Can you work these out from the model? Positions are in its coordinate system, mm. Face numbers are marked on the shaded views. Coordinates: 2 decimals unless noted, no trailing zeros. Write each loop counter-clockwise with the first axis right and the second up, starting at its lowest first coordinate (ties: lowest second). Pieces come first, ordered by that corner, then holes. Notation, with made-up numbers: M -26,84 L 8,84 A8 cw 8,89 Z; hole C -13.75,53 d1. An arc over 180 degrees is marked long. Use one line per item in the form item = value. Start each with the question number.
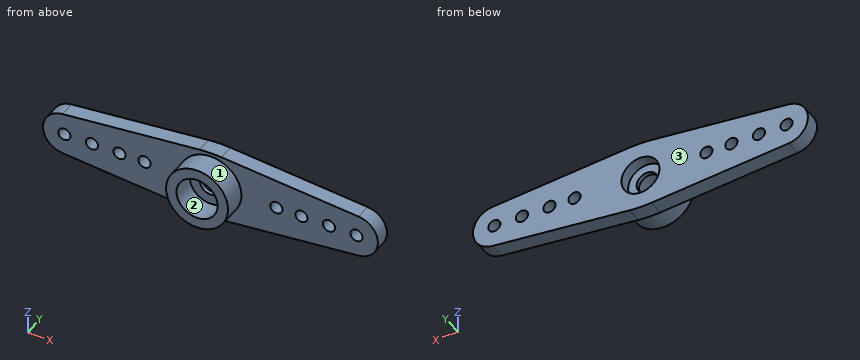
```python
from build123d import *

# Parameters (mm, degrees)
SKETCH1_R           = 3.3655
SKETCH1_R_2         = 2.2352
BOSS_EXTRUDE1_DEPTH = 2.54
SKETCH2_R           = 0.6604
SKETCH2_R_2         = 2.31775
SKETCH2_R_3         = 3.3655
SKETCH2_R_4         = 2.2352
SKETCH2_R_5         = 1.143
BOSS_EXTRUDE2_DEPTH = 1.7272
FILLET1_R           = 12.7
CUT_EXTRUDE1_START  = -1.27
SKETCH3_R           = 2.06375
SKETCH3_R_2         = 1.143
CUT_EXTRUDE1_DEPTH  = 1.27
SCALE1_SCALE        = 1.483924155


with BuildPart() as part:
    # Sketch1 → Boss-Extrude1 (new body)
    with BuildSketch(Plane(origin=(0, 0, 0), x_dir=(1, 0, 0), z_dir=(0, 1, 0))):
        with Locations(Location((0, 0, 0), (0, 0, 270))):
            Circle(SKETCH1_R)
        with Locations(Location((0, 0, 0), (0, 0, 270))):
            Circle(SKETCH1_R_2, mode=Mode.SUBTRACT)
    extrude(amount=BOSS_EXTRUDE1_DEPTH)

    # Sketch2 → Boss-Extrude2 (add)
    # profile 1 of 7: a face of its own
    with BuildSketch(Plane(origin=(0, 2.54, 0), x_dir=(1, 0, 0), z_dir=(0, 1, 0))):
        with BuildLine():
            ThreePointArc((-0.713521748, -3.755518873), (-3.8227, 0), (-0.713521748, 3.755518873))
            Line((-0.713521748, 3.755518873), (-16.092265178, 2.307544345))
            ThreePointArc((-16.092265178, 2.307544345), (-14.314807913, 1.713991165), (-13.55725, 0))
            ThreePointArc((-13.55725, 0), (-14.314807913, -1.713991165), (-16.092265178, -2.307544345))
            Line((-16.092265178, -2.307544345), (-0.713521748, -3.755518873))
        make_face()
        with Locations(Location((-12.8778, 0, 0), (0, 0, 270))):
            Circle(SKETCH2_R, mode=Mode.SUBTRACT)
        with Locations(Location((-9.8806, 0, 0), (0, 0, 270))):
            Circle(SKETCH2_R, mode=Mode.SUBTRACT)
        with Locations(Location((-7.1628, 0, 0), (0, 0, 270))):
            Circle(SKETCH2_R, mode=Mode.SUBTRACT)
    # profile 2 of 7: a face of its own
    with BuildSketch(Plane(origin=(0, 2.54, 0), x_dir=(1, 0, 0), z_dir=(0, 1, 0))):
        with Locations((-15.875, 0)):
            Circle(SKETCH2_R_2)
        with Locations(Location((-15.875, 0, 0), (0, 0, 270))):
            Circle(SKETCH2_R, mode=Mode.SUBTRACT)
    # profile 3 of 7: a face of its own
    with BuildSketch(Plane(origin=(0, 2.54, 0), x_dir=(1, 0, 0), z_dir=(0, 1, 0))):
        with BuildLine():
            Line((16.092265178, 2.307544345), (0.713521748, 3.755518873))
            ThreePointArc((0.713521748, 3.755518873), (2.944538578, 2.437771083), (3.8227, 0))
            ThreePointArc((3.8227, 0), (2.944538578, -2.437771083), (0.713521748, -3.755518873))
            Line((0.713521748, -3.755518873), (16.092265178, -2.307544345))
            ThreePointArc((16.092265178, -2.307544345), (13.55725, 0), (16.092265178, 2.307544345))
        make_face()
        with Locations(Location((7.1628, 0, 0), (0, 0, 270))):
            Circle(SKETCH2_R, mode=Mode.SUBTRACT)
        with Locations(Location((9.8806, 0, 0), (0, 0, 270))):
            Circle(SKETCH2_R, mode=Mode.SUBTRACT)
        with Locations(Location((12.8778, 0, 0), (0, 0, 270))):
            Circle(SKETCH2_R, mode=Mode.SUBTRACT)
    # profile 4 of 7: a face of its own
    with BuildSketch(Plane(origin=(0, 2.54, 0), x_dir=(1, 0, 0), z_dir=(0, 1, 0))):
        with Locations((15.875, 0)):
            Circle(SKETCH2_R_2)
        with Locations(Location((15.875, 0, 0), (0, 0, 270))):
            Circle(SKETCH2_R, mode=Mode.SUBTRACT)
    # profile 5 of 7: a face of its own
    with BuildSketch(Plane(origin=(0, 2.54, 0), x_dir=(1, 0, 0), z_dir=(0, 1, 0))):
        with BuildLine():
            Line((0.713521748, 3.755518873), (0, 3.8227))
            Line((0, 3.8227), (-0.713521748, 3.755518873))
            ThreePointArc((-0.713521748, 3.755518873), (-3.8227, 0), (-0.713521748, -3.755518873))
            Line((-0.713521748, -3.755518873), (0, -3.8227))
            Line((0, -3.8227), (0.713521748, -3.755518873))
            ThreePointArc((0.713521748, -3.755518873), (2.944538578, -2.437771083), (3.8227, 0))
            ThreePointArc((3.8227, 0), (2.944538578, 2.437771083), (0.713521748, 3.755518873))
        make_face()
        with Locations(Location((0, 0, 0), (0, 0, 270))):
            Circle(SKETCH2_R_3, mode=Mode.SUBTRACT)
    # profile 6 of 7: a face of its own
    with BuildSketch(Plane(origin=(0, 2.54, 0), x_dir=(1, 0, 0), z_dir=(0, 1, 0))):
        with Locations(Location((0, 0, 0), (0, 0, 270))):
            Circle(SKETCH2_R_3)
        with Locations(Location((0, 0, 0), (0, 0, 270))):
            Circle(SKETCH2_R_4, mode=Mode.SUBTRACT)
    # profile 7 of 7: a face of its own
    with BuildSketch(Plane(origin=(0, 2.54, 0), x_dir=(1, 0, 0), z_dir=(0, 1, 0))):
        with Locations(Location((0, 0, 0), (0, 0, 270))):
            Circle(SKETCH2_R_4)
        with Locations(Location((0, 0, 0), (0, 0, 270))):
            Circle(SKETCH2_R_5, mode=Mode.SUBTRACT)
    extrude(amount=BOSS_EXTRUDE2_DEPTH)

    # Fillet1
    fillet1_edges = [part.edges().sort_by_distance(p)[0] for p in [
        (0, 3.4036, -3.8227),
        (0, 3.4036, 3.8227),
    ]]
    fillet(fillet1_edges, radius=FILLET1_R)

    # Sketch3 → Cut-Extrude1 (cut)
    with BuildSketch(Plane(origin=(0, 4.2672, 0), x_dir=(1, 0, 0), z_dir=(0, 1, 0)).offset(CUT_EXTRUDE1_START)):
        with Locations(Location((0, 0, 0), (0, 0, 270))):
            Circle(SKETCH3_R)
        with Locations(Location((0, 0, 0), (0, 0, 270))):
            Circle(SKETCH3_R_2, mode=Mode.SUBTRACT)
    extrude(amount=CUT_EXTRUDE1_DEPTH, mode=Mode.SUBTRACT)


with BuildPart() as part_1:
    # Scale1: scaled about (0, 3.112125365, 0)
    add(part.part.scale(SCALE1_SCALE).moved(Location((0, -1.506032637, 0))))


solid = part_1.part
```
1) If we mould it in two halves opening along X, with no side actions, what happens to the marked faces 1, 2 and 3? For each: +X half, -X half, draft (parallel to the pull), parting line (faces both ways), or undercut.
2) Will these pins go through, and if not, where does the flat tip stop? pin 1 Ø2.5 at (x, z) = (-23.56, 0) entering from -Y; pin 2 Ø4 at (x, z) = (-19.5, -0.5) entering from +Y; pin 3 Ø1.2 at (x, z) = (14.66, 0) entering from +Y; pin 4 Ø5.5 at (x, z) = (0, 0) entering from +Y.
3) Suppose I cut it at C-C on x = -16.5. Please give me the cut outline in (y, z).
4) Please list where these lines run through material, in increasing order: line 1 (Y direction, x = -16, z = 0.5); line 2 (Y direction, x = -2.5, z = -1.5); line 3 (Z direction, x = -15, y = 4.25).
5) Suppose I cut it at A-A on z = 0. State how many separate pieces and enclosed holes the cut face has, and give its area (3 significant figures).
Computed values:
q1.face_1 = parting line
q1.face_2 = undercut
q1.face_3 = draft
q2.pin_1 = 2.26
q2.pin_2 = 4.83
q2.pin_3 = through
q2.pin_4 = 2.94
q3.outline = M 2.26,-4.12 L 4.83,-4.12 L 4.83,4.12 L 2.26,4.12 Z
q4.line_1 = 2.26 to 4.83
q4.line_2 = 2.26 to 2.94
q4.line_3 = -4.26 to -0.92, 0.92 to 4.26
q5.separate_pieces = 10
q5.enclosed_holes = 0
q5.area = 97.0 mm²
